```python
from build123d import *

# Parameters (mm, degrees)
SKETCH_1_R      = 1.7
SKETCH_1_R_2    = 2
SKETCH_1_R_3    = 2.5
EXTRUDE_2_DEPTH = 4


with BuildPart() as part:
    # 草图1 → 凸台-拉伸2 (new body)
    with BuildSketch(Plane(origin=(0, 0, 0), x_dir=(1, 0, 0), z_dir=(0, 1, 0))):
        with BuildLine():
            Line((60, 160), (0, 160))
            Line((0, 160), (-60, 160))
            ThreePointArc((-60, 160), (-67.071067812, 157.071067812), (-70, 150))
            Line((-70, 150), (-70, 0))
            Line((-70, 0), (-70, -150))
            ThreePointArc((-70, -150), (-67.071067812, -157.071067812), (-60, -160))
            Line((-60, -160), (60, -160))
            ThreePointArc((60, -160), (67.071067812, -157.071067812), (70, -150))
            Line((70, -150), (70, 150))
            ThreePointArc((70, 150), (67.071067812, 157.071067812), (60, 160))
        make_face()
        with Locations(Location((-62, 132, 0), (0, 0, 270))):
            Circle(SKETCH_1_R, mode=Mode.SUBTRACT)
        with Locations(Location((-62, -148, 0), (0, 0, 270))):
            Circle(SKETCH_1_R, mode=Mode.SUBTRACT)
        with Locations(Location((-48, -148, 0), (0, 0, 270))):
            Circle(SKETCH_1_R, mode=Mode.SUBTRACT)
        with Locations(Location((-62, -132, 0), (0, 0, 270))):
            Circle(SKETCH_1_R, mode=Mode.SUBTRACT)
        with Locations(Location((-60, -120, 0), (0, 0, 270))):
            Circle(SKETCH_1_R_2, mode=Mode.SUBTRACT)
        with Locations(Location((-48, -132, 0), (0, 0, 270))):
            Circle(SKETCH_1_R, mode=Mode.SUBTRACT)
        with Locations(Location((-35, -150, 0), (0, 0, 270))):
            Circle(SKETCH_1_R_3, mode=Mode.SUBTRACT)
        with Locations(Location((-40, -120, 0), (0, 0, 270))):
            Circle(SKETCH_1_R_2, mode=Mode.SUBTRACT)
        with Locations(Location((-60, -100, 0), (0, 0, 270))):
            Circle(SKETCH_1_R_2, mode=Mode.SUBTRACT)
        with Locations(Location((-60, -80, 0), (0, 0, 270))):
            Circle(SKETCH_1_R_2, mode=Mode.SUBTRACT)
        with Locations(Location((-40, -100, 0), (0, 0, 270))):
            Circle(SKETCH_1_R_2, mode=Mode.SUBTRACT)
        with Locations(Location((-40, -80, 0), (0, 0, 270))):
            Circle(SKETCH_1_R_2, mode=Mode.SUBTRACT)
        with Locations(Location((-20, -120, 0), (0, 0, 270))):
            Circle(SKETCH_1_R_2, mode=Mode.SUBTRACT)
        with BuildLine():
            ThreePointArc((15, -125), (22.071067812, -127.928932188), (25, -135))
            Line((25, -135), (25, -145))
            ThreePointArc((25, -145), (22.071067812, -152.071067812), (15, -155))
            Line((15, -155), (-15, -155))
            ThreePointArc((-15, -155), (-22.071067812, -152.071067812), (-25, -145))
            Line((-25, -145), (-25, -135))
            ThreePointArc((-25, -135), (-22.071067812, -127.928932188), (-15, -125))
            Line((-15, -125), (15, -125))
        make_face(mode=Mode.SUBTRACT)
        with Locations(Location((0, -120, 0), (0, 0, 270))):
            Circle(SKETCH_1_R_2, mode=Mode.SUBTRACT)
        with Locations(Location((-20, -100, 0), (0, 0, 270))):
            Circle(SKETCH_1_R_2, mode=Mode.SUBTRACT)
        with Locations(Location((-20, -80, 0), (0, 0, 270))):
            Circle(SKETCH_1_R_2, mode=Mode.SUBTRACT)
        with Locations(Location((0, -100, 0), (0, 0, 270))):
            Circle(SKETCH_1_R_2, mode=Mode.SUBTRACT)
        with Locations(Location((0, -80, 0), (0, 0, 270))):
            Circle(SKETCH_1_R_2, mode=Mode.SUBTRACT)
        with Locations(Location((-60, -60, 0), (0, 0, 270))):
            Circle(SKETCH_1_R_2, mode=Mode.SUBTRACT)
        with Locations(Location((-60, -40, 0), (0, 0, 270))):
            Circle(SKETCH_1_R_2, mode=Mode.SUBTRACT)
        with Locations(Location((-40, -60, 0), (0, 0, 270))):
            Circle(SKETCH_1_R_2, mode=Mode.SUBTRACT)
        with Locations(Location((-40, -40, 0), (0, 0, 270))):
            Circle(SKETCH_1_R_2, mode=Mode.SUBTRACT)
        with Locations(Location((-60, -20, 0), (0, 0, 270))):
            Circle(SKETCH_1_R_2, mode=Mode.SUBTRACT)
        with Locations(Location((-40, -20, 0), (0, 0, 270))):
            Circle(SKETCH_1_R_2, mode=Mode.SUBTRACT)
        with Locations(Location((-20, -60, 0), (0, 0, 270))):
            Circle(SKETCH_1_R_2, mode=Mode.SUBTRACT)
        with Locations(Location((-20, -40, 0), (0, 0, 270))):
            Circle(SKETCH_1_R_2, mode=Mode.SUBTRACT)
        with Locations(Location((0, -60, 0), (0, 0, 270))):
            Circle(SKETCH_1_R_2, mode=Mode.SUBTRACT)
        with Locations(Location((0, -40, 0), (0, 0, 270))):
            Circle(SKETCH_1_R_2, mode=Mode.SUBTRACT)
        with Locations(Location((-20, -20, 0), (0, 0, 270))):
            Circle(SKETCH_1_R_2, mode=Mode.SUBTRACT)
        with Locations(Location((0, -20, 0), (0, 0, 270))):
            Circle(SKETCH_1_R_2, mode=Mode.SUBTRACT)
        with Locations(Location((20, -120, 0), (0, 0, 270))):
            Circle(SKETCH_1_R_2, mode=Mode.SUBTRACT)
        with Locations(Location((20, -100, 0), (0, 0, 270))):
            Circle(SKETCH_1_R_2, mode=Mode.SUBTRACT)
        with Locations(Location((20, -80, 0), (0, 0, 270))):
            Circle(SKETCH_1_R_2, mode=Mode.SUBTRACT)
        with Locations(Location((35, -150, 0), (0, 0, 270))):
            Circle(SKETCH_1_R_3, mode=Mode.SUBTRACT)
        with Locations(Location((40, -120, 0), (0, 0, 270))):
            Circle(SKETCH_1_R_2, mode=Mode.SUBTRACT)
        with Locations(Location((48, -148, 0), (0, 0, 270))):
            Circle(SKETCH_1_R, mode=Mode.SUBTRACT)
        with Locations(Location((62, -148, 0), (0, 0, 270))):
            Circle(SKETCH_1_R, mode=Mode.SUBTRACT)
        with Locations(Location((48, -132, 0), (0, 0, 270))):
            Circle(SKETCH_1_R, mode=Mode.SUBTRACT)
        with Locations(Location((62, -132, 0), (0, 0, 270))):
            Circle(SKETCH_1_R, mode=Mode.SUBTRACT)
        with Locations(Location((60, -120, 0), (0, 0, 270))):
            Circle(SKETCH_1_R_2, mode=Mode.SUBTRACT)
        with Locations(Location((40, -100, 0), (0, 0, 270))):
            Circle(SKETCH_1_R_2, mode=Mode.SUBTRACT)
        with Locations(Location((40, -80, 0), (0, 0, 270))):
            Circle(SKETCH_1_R_2, mode=Mode.SUBTRACT)
        with Locations(Location((60, -100, 0), (0, 0, 270))):
            Circle(SKETCH_1_R_2, mode=Mode.SUBTRACT)
        with Locations(Location((60, -80, 0), (0, 0, 270))):
            Circle(SKETCH_1_R_2, mode=Mode.SUBTRACT)
        with Locations(Location((20, -60, 0), (0, 0, 270))):
            Circle(SKETCH_1_R_2, mode=Mode.SUBTRACT)
        with Locations(Location((20, -40, 0), (0, 0, 270))):
            Circle(SKETCH_1_R_2, mode=Mode.SUBTRACT)
        with Locations(Location((20, -20, 0), (0, 0, 270))):
            Circle(SKETCH_1_R_2, mode=Mode.SUBTRACT)
        with Locations(Location((40, -60, 0), (0, 0, 270))):
            Circle(SKETCH_1_R_2, mode=Mode.SUBTRACT)
        with Locations(Location((40, -40, 0), (0, 0, 270))):
            Circle(SKETCH_1_R_2, mode=Mode.SUBTRACT)
        with Locations(Location((60, -60, 0), (0, 0, 270))):
            Circle(SKETCH_1_R_2, mode=Mode.SUBTRACT)
        with Locations(Location((60, -40, 0), (0, 0, 270))):
            Circle(SKETCH_1_R_2, mode=Mode.SUBTRACT)
        with Locations(Location((40, -20, 0), (0, 0, 270))):
            Circle(SKETCH_1_R_2, mode=Mode.SUBTRACT)
        with Locations(Location((60, -20, 0), (0, 0, 270))):
            Circle(SKETCH_1_R_2, mode=Mode.SUBTRACT)
        with Locations(Location((-60, 20, 0), (0, 0, 270))):
            Circle(SKETCH_1_R_2, mode=Mode.SUBTRACT)
        with Locations(Location((-40, 20, 0), (0, 0, 270))):
            Circle(SKETCH_1_R_2, mode=Mode.SUBTRACT)
        with Locations(Location((-60, 40, 0), (0, 0, 270))):
            Circle(SKETCH_1_R_2, mode=Mode.SUBTRACT)
        with Locations(Location((-60, 60, 0), (0, 0, 270))):
            Circle(SKETCH_1_R_2, mode=Mode.SUBTRACT)
        with Locations(Location((-40, 40, 0), (0, 0, 270))):
            Circle(SKETCH_1_R_2, mode=Mode.SUBTRACT)
        with Locations(Location((-40, 60, 0), (0, 0, 270))):
            Circle(SKETCH_1_R_2, mode=Mode.SUBTRACT)
        with Locations(Location((-20, 20, 0), (0, 0, 270))):
            Circle(SKETCH_1_R_2, mode=Mode.SUBTRACT)
        with Locations(Location((0, 20, 0), (0, 0, 270))):
            Circle(SKETCH_1_R_2, mode=Mode.SUBTRACT)
        with Locations(Location((-20, 40, 0), (0, 0, 270))):
            Circle(SKETCH_1_R_2, mode=Mode.SUBTRACT)
        with Locations(Location((-20, 60, 0), (0, 0, 270))):
            Circle(SKETCH_1_R_2, mode=Mode.SUBTRACT)
        with Locations(Location((0, 40, 0), (0, 0, 270))):
            Circle(SKETCH_1_R_2, mode=Mode.SUBTRACT)
        with Locations(Location((0, 60, 0), (0, 0, 270))):
            Circle(SKETCH_1_R_2, mode=Mode.SUBTRACT)
        with Locations(Location((-60, 80, 0), (0, 0, 270))):
            Circle(SKETCH_1_R_2, mode=Mode.SUBTRACT)
        with Locations(Location((-60, 100, 0), (0, 0, 270))):
            Circle(SKETCH_1_R_2, mode=Mode.SUBTRACT)
        with Locations(Location((-40, 80, 0), (0, 0, 270))):
            Circle(SKETCH_1_R_2, mode=Mode.SUBTRACT)
        with Locations(Location((-40, 100, 0), (0, 0, 270))):
            Circle(SKETCH_1_R_2, mode=Mode.SUBTRACT)
        with Locations(Location((-60, 120, 0), (0, 0, 270))):
            Circle(SKETCH_1_R_2, mode=Mode.SUBTRACT)
        with Locations(Location((-48, 132, 0), (0, 0, 270))):
            Circle(SKETCH_1_R, mode=Mode.SUBTRACT)
        with Locations(Location((-62, 138, 0), (0, 0, 270))):
            Circle(SKETCH_1_R, mode=Mode.SUBTRACT)
        with Locations(Location((-48, 138, 0), (0, 0, 270))):
            Circle(SKETCH_1_R, mode=Mode.SUBTRACT)
        with Locations(Location((-40, 120, 0), (0, 0, 270))):
            Circle(SKETCH_1_R_2, mode=Mode.SUBTRACT)
        with Locations(Location((-35, 150, 0), (0, 0, 270))):
            Circle(SKETCH_1_R_3, mode=Mode.SUBTRACT)
        with Locations(Location((-20, 80, 0), (0, 0, 270))):
            Circle(SKETCH_1_R_2, mode=Mode.SUBTRACT)
        with Locations(Location((-20, 100, 0), (0, 0, 270))):
            Circle(SKETCH_1_R_2, mode=Mode.SUBTRACT)
        with Locations(Location((0, 80, 0), (0, 0, 270))):
            Circle(SKETCH_1_R_2, mode=Mode.SUBTRACT)
        with Locations(Location((0, 100, 0), (0, 0, 270))):
            Circle(SKETCH_1_R_2, mode=Mode.SUBTRACT)
        with Locations(Location((-20, 120, 0), (0, 0, 270))):
            Circle(SKETCH_1_R_2, mode=Mode.SUBTRACT)
        with Locations(Location((0, 120, 0), (0, 0, 270))):
            Circle(SKETCH_1_R_2, mode=Mode.SUBTRACT)
        with BuildLine():
            Line((-15, 155), (0, 155))
            Line((0, 155), (15, 155))
            ThreePointArc((15, 155), (22.071067812, 152.071067812), (25, 145))
            Line((25, 145), (25, 135))
            ThreePointArc((25, 135), (22.071067812, 127.928932188), (15, 125))
            Line((15, 125), (-15, 125))
            ThreePointArc((-15, 125), (-22.071067812, 127.928932188), (-25, 135))
            Line((-25, 135), (-25, 145))
            ThreePointArc((-25, 145), (-22.071067812, 152.071067812), (-15, 155))
        make_face(mode=Mode.SUBTRACT)
        with Locations(Location((20, 20, 0), (0, 0, 270))):
            Circle(SKETCH_1_R_2, mode=Mode.SUBTRACT)
        with Locations(Location((20, 40, 0), (0, 0, 270))):
            Circle(SKETCH_1_R_2, mode=Mode.SUBTRACT)
        with Locations(Location((20, 60, 0), (0, 0, 270))):
            Circle(SKETCH_1_R_2, mode=Mode.SUBTRACT)
        with Locations(Location((40, 20, 0), (0, 0, 270))):
            Circle(SKETCH_1_R_2, mode=Mode.SUBTRACT)
        with Locations(Location((60, 20, 0), (0, 0, 270))):
            Circle(SKETCH_1_R_2, mode=Mode.SUBTRACT)
        with Locations(Location((40, 40, 0), (0, 0, 270))):
            Circle(SKETCH_1_R_2, mode=Mode.SUBTRACT)
        with Locations(Location((40, 60, 0), (0, 0, 270))):
            Circle(SKETCH_1_R_2, mode=Mode.SUBTRACT)
        with Locations(Location((60, 40, 0), (0, 0, 270))):
            Circle(SKETCH_1_R_2, mode=Mode.SUBTRACT)
        with Locations(Location((60, 60, 0), (0, 0, 270))):
            Circle(SKETCH_1_R_2, mode=Mode.SUBTRACT)
        with Locations(Location((20, 80, 0), (0, 0, 270))):
            Circle(SKETCH_1_R_2, mode=Mode.SUBTRACT)
        with Locations(Location((20, 100, 0), (0, 0, 270))):
            Circle(SKETCH_1_R_2, mode=Mode.SUBTRACT)
        with Locations(Location((20, 120, 0), (0, 0, 270))):
            Circle(SKETCH_1_R_2, mode=Mode.SUBTRACT)
        with Locations(Location((40, 80, 0), (0, 0, 270))):
            Circle(SKETCH_1_R_2, mode=Mode.SUBTRACT)
        with Locations(Location((40, 100, 0), (0, 0, 270))):
            Circle(SKETCH_1_R_2, mode=Mode.SUBTRACT)
        with Locations(Location((60, 80, 0), (0, 0, 270))):
            Circle(SKETCH_1_R_2, mode=Mode.SUBTRACT)
        with Locations(Location((60, 100, 0), (0, 0, 270))):
            Circle(SKETCH_1_R_2, mode=Mode.SUBTRACT)
        with Locations(Location((40, 120, 0), (0, 0, 270))):
            Circle(SKETCH_1_R_2, mode=Mode.SUBTRACT)
        with Locations(Location((35, 150, 0), (0, 0, 270))):
            Circle(SKETCH_1_R_3, mode=Mode.SUBTRACT)
        with Locations(Location((48, 132, 0), (0, 0, 270))):
            Circle(SKETCH_1_R, mode=Mode.SUBTRACT)
        with Locations(Location((60, 120, 0), (0, 0, 270))):
            Circle(SKETCH_1_R_2, mode=Mode.SUBTRACT)
        with Locations(Location((62, 132, 0), (0, 0, 270))):
            Circle(SKETCH_1_R, mode=Mode.SUBTRACT)
        with Locations(Location((48, 148, 0), (0, 0, 270))):
            Circle(SKETCH_1_R, mode=Mode.SUBTRACT)
        with Locations(Location((62, 148, 0), (0, 0, 270))):
            Circle(SKETCH_1_R, mode=Mode.SUBTRACT)
    extrude(amount=EXTRUDE_2_DEPTH)


solid = part.part
```
Check sheet for the modelled part. Datum: model origin and axes. Units: mm. A direction names the side the tool comes from. Coordinates: 2 decimals unless noted, no trailing zeros.
1) Sectioned sample at A-A (y = 1.5). Count the separate pieces of the cut face and the enclosed holes in it, and give its area (3 significant figures).
2) Release check for a two-part mould opening along Z. For faces 3 (the face through (-22.15, 1.97, 128.01)), 4 (the face through (67.15, 1.97, -156.99)), 5 (the face through (-1, 4, -2)) record: released by +Z, released by -Z, zero draft, split by the parting line, or undercut.
3) Material ranges on probe 1 along Z at (x, y) = (-23, 1.9); probe 2 along Z at (x, y) = (8, 0.8); probe 3 along Z at (x, y) = (-46.5, 3.35), recorded low to high.
4) Gauge pin test, flat end, axial feed: pin 1 (2.5 mm diameter, centred on x = -20, z = 20, fed in from -Y). Record the tip position at first contact, or that the pin passes through.
5) Access from +Z, -Z, +X, -X, +Y, -Y to the whole of each face (thin tool, end or side, straight path). Record for faces 1 (the face through (66.99, 1.97, 157.15)), 2 (the face through (22.15, 1.97, -128.01)).
Check sheet entries:
1. separate pieces: 1
1. enclosed holes: 106
1. area: 40,600 mm2
2. face 3: undercut
2. face 4: released by -Z
2. face 5: zero draft
3. probe 1: z = -160 to -151, -129 to 129, 151 to 160
3. probe 2: z = -160 to -155, -125 to 125, 155 to 160
3. probe 3: z = -160 to -138.8, -137.2 to -132.8, -131.2 to 131.2, 132.8 to 147.2, 148.8 to 160
4. pin 1: passes through
5. face 1: +Z, +X, +Y, -Y
5. face 2: +Y, -Y
